```python
from build123d import *

# Parameters (mm, degrees)
BOSS_EXTRUDE1_DEPTH = 3.4036


with BuildPart() as part:
    # Sketch1 → Boss-Extrude1 (new body)
    with BuildSketch(Plane.XY):
        Polygon((8689.636759917, 2979.750055989), (8587.64819291, 2974.720855989), (8587.64819291, 2962.020855989), (8593.99819291, 2962.020855989), (8593.99819291, 2916.453255989), (8587.64819291, 2916.453255989), (8587.64819291, 2903.753255989), (8689.636759917, 2898.724055989), (8689.636759917, 2911.424055989), (8682.89819291, 2911.424055989), (8682.89819291, 2967.050055989), (8689.636759917, 2967.050055989), align=None)
        with BuildLine():
            Line((8606.69819291, 2952.495855989), (8606.69819291, 2925.978255989))
            ThreePointArc((8606.69819291, 2925.978255989), (8608.55806485, 2921.488127929), (8613.04819291, 2919.628255989))
            Line((8613.04819291, 2919.628255989), (8663.84819291, 2919.628255989))
            ThreePointArc((8663.84819291, 2919.628255989), (8668.338320971, 2921.488127929), (8670.19819291, 2925.978255989))
            Line((8670.19819291, 2925.978255989), (8670.19819291, 2952.495855989))
            ThreePointArc((8670.19819291, 2952.495855989), (8668.338320971, 2956.98598405), (8663.84819291, 2958.845855989))
            Line((8663.84819291, 2958.845855989), (8613.04819291, 2958.845855989))
            ThreePointArc((8613.04819291, 2958.845855989), (8608.55806485, 2956.98598405), (8606.69819291, 2952.495855989))
        make_face(mode=Mode.SUBTRACT)
    extrude(amount=BOSS_EXTRUDE1_DEPTH)


solid = part.part
```
Geometry: final body of the model. Coordinates: model frame, mm. A direction names the side the tool comes from. Coordinates: 2 decimals unless noted, no trailing zeros. Order: outer loops, then holes, each group sorted by start corner. A loop starts at its lowest first (then second) coordinate and runs counter-clockwise, first axis right, second up. Notation, with made-up numbers: (8, 3) - (64, 3) arc R37 cw to (64, 42) - close; hole circle Ø5 at (52.5, 85). An arc over 180 degrees is marked (long way). Write each question's results on one line, items separated by ' | '.
(1) Section query A-A, the plane z = 2.65. Return the cut outline in (x, y), plus the area to 3 significant figures.
Values found:
outline: (8587.65, 2903.75) - (8689.64, 2898.72) - (8689.64, 2911.42) - (8682.9, 2911.42) - (8682.9, 2967.05) - (8689.64, 2967.05) - (8689.64, 2979.75) - (8587.65, 2974.72) - (8587.65, 2962.02) - (8594, 2962.02) - (8594, 2916.45) - (8587.65, 2916.45) - close; hole (8606.7, 2925.98) arc R6.35 ccw to (8613.05, 2919.63) - (8663.85, 2919.63) arc R6.35 ccw to (8670.2, 2925.98) - (8670.2, 2952.5) arc R6.35 ccw to (8663.85, 2958.85) - (8613.05, 2958.85) arc R6.35 ccw to (8606.7, 2952.5) - close | area: 4,630 mm²
(2) First-contact query: pin 1 Ø1.7 at (x, z) = (8628, 1.5) entering from -Y; pin 2 Ø1.7 at (y, z) = (2938, 1.5) entering from +X; pin 3 Ø1.7 at (x, z) = (8591, 2) entering from +Y. Flat tips, straight axial feed; report the tip coordinate or a pass-through.
Values found:
pin 1: stops at y = 2901.72 | pin 2: stops at x = 8682.9 | pin 3: stops at y = 2974.93
(3) Set-up query: faces 4 (the face through (8638, 2913, 3.404)), 5 (the face through (8639.36, 2977.27, 1.68)), 6 (the face through (8682.898, 2939, 2)), 7 (the face through (8638, 2919.628, 2)), 8 (the face through (8593.998, 2940, 2)). Return all of +Z, -Z, +X, -X, +Y, -Y with unobstructed straight access to the full face (end or side cutting, diameter ignored); none if empty.
Values found:
face 4: +Z, +X, -X, +Y, -Y | face 5: +Z, -Z, -X, +Y | face 6: +Z, -Z, +X | face 7: +Z, -Z | face 8: +Z, -Z, -X
(4) Line query: line 1 (X direction, y = 2930, z = 2.35); line 2 (Y direction, x = 8592, z = 2.7); line 3 (Y direction, x = 8659.5, z = 0.2). Output: solid intervals per line, ascending. Write a range as [from, to].
Values found:
line 1: x = [8594, 8606.7], [8670.2, 8682.9] | line 2: y = [2903.54, 2916.45], [2962.02, 2974.94] | line 3: y = [2900.21, 2919.63], [2958.85, 2978.26]
(5) Section query D-D, the plane y = 2964.5. Return the cut outline in (x, z), plus the area to 3 significant figures.
Values found:
outline: (8587.65, 0) - (8682.9, 0) - (8682.9, 3.4) - (8587.65, 3.4) - close | area: 324 mm²
(6) Section query B-B, the plane y = 2934.5. Return the cut outline in (x, z).
Values found:
outline: (8594, 0) - (8606.7, 0) - (8606.7, 3.4) - (8594, 3.4) - close; (8670.2, 0) - (8682.9, 0) - (8682.9, 3.4) - (8670.2, 3.4) - close
(7) Section query C-C, the plane x = 8667. Return the cut outline in (y, z).
Values found:
outline: (2899.84, 0) - (2920.47, 0) - (2920.47, 3.4) - (2899.84, 3.4) - close; (2958.01, 0) - (2978.63, 0) - (2978.63, 3.4) - (2958.01, 3.4) - close
(8) Mould query, pull axis X, two halves, no side actions, for faces 1 (the face through (8587.648, 2910, 2)), 2 (the face through (8591, 2962.021, 2)), 3 (the face through (8639, 2958.846, 2)). Classes: +X half, -X half, draft (parallel to the pull), parting line (faces both ways), or undercut.
Values found:
face 1: -X half | face 2: draft | face 3: undercut
